Build history of the part. All positions in model axes, mm. Face numbers are marked on the shaded views. Round coordinates to 2 decimals unless told otherwise and drop trailing zeros. Order: outer loops, then holes, each group sorted by start corner. A loop starts at its lowest first (then second) coordinate and runs counter-clockwise, first axis right, second up. Notation, with made-up numbers: (26.5, 0.5) -> (51.5, 0.5) arc R23 ccw to (51.5, 26.5) -> close; hole circle Ø5 at (37.5, 86). An arc over 180 degrees is marked (long way). Use a Markdown table: item, result. Add a question column.
Item 1: Slice it at A-A, the plane z = 0. Give the cut face in (x, y).
Item 2: Probe L1, parallel to Y at x = 30, z = 0; L2, parallel to X at y = -36.5, z = -18; L3, parallel to Z at x = 4, y = -23. List the from-to ranges inside material, lowest first.
Item 3: Two-plate mould, pull along Y, no slides. Class the marked faces 1 and 2: released by +Y, released by -Y, zero draft, split by the parting line, or undercut.
Item 4: Slice it at B-B, the plane y = -29.5. Give the cut face in (x, z), plus the area to 3 significant figures.
Item 5: Pin check, flat tips, straight feed: pin 1 (8 mm diameter, centred on x = 52, y = 28, fed in from +Z); pin 2 (3 mm diameter, centred on x = 39, y = -27, fed in from +Z); pin 3 (6 mm diameter, centred on x = 82, y = -12.5, fed in from +Z); pin 4 (1.5 mm diameter, centred on x = 43.5, y = 32, fed in from -Z). Stop position of each tip, or through.
Item 6: Slice it at C-C, the plane x = 38. Give the cut face in (y, z), plus the area to 3 significant figures.
Item 7: Slice it at D-D, the plane y = 18. Give the cut face in (x, z).
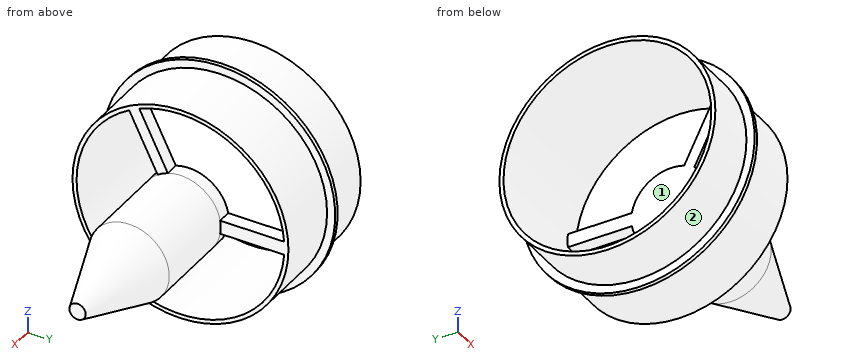
from build123d import *
from build123d.topology import SkipClean

# Parameters (mm, degrees)
SKETCH_1_R          = 39.7
EXTRUDE_1_DEPTH     = 45
SKETCH_2_R          = 38.2
CUT_EXTRUDE_1_DEPTH = 72.952623302
SKETCH_3_R          = 42.7
SKETCH_3_R_2        = 39.7
EXTRUDE_2_DEPTH     = 1.5
EXTRUDE_START       = -5
EXTRUDE_3_DEPTH     = 5
SKETCH_7_R          = 14.8
EXTRUDE_4_DEPTH     = 32.1
SKETCH_9_R          = 14.8
SKETCH_10_R         = 3


with BuildPart() as part:
    # Эскиз1 → Бобышка-Вытянуть1 (new body)
    with BuildSketch(Plane(origin=(0, 0, 0), x_dir=(0, 0, -1), z_dir=(1, 0, 0))):
        with Locations(Location((0, 0, 0), (0, 0, 180))):
            Circle(SKETCH_1_R)
    extrude(amount=EXTRUDE_1_DEPTH)

    # Эскиз2 → Вырез-Вытянуть1 (cut, through all)
    with BuildSketch(Plane.ZY):
        Circle(SKETCH_2_R)
    extrude(amount=-CUT_EXTRUDE_1_DEPTH, mode=Mode.SUBTRACT)

    # Эскиз3 → Бобышка-Вытянуть2 (add)
    with BuildSketch(Plane(origin=(19.4, 0, 0), x_dir=(0, 0, -1), z_dir=(1, 0, 0))):
        Circle(SKETCH_3_R)
        with Locations(Location((0, 0, 0), (0, 0, 180))):
            Circle(SKETCH_3_R_2, mode=Mode.SUBTRACT)
    extrude(amount=EXTRUDE_2_DEPTH)

    # Эскиз6 → Бобышка-Вытянуть3 (add)
    with BuildSketch(Plane(origin=(45, 0, 0), x_dir=(0, 0, -1), z_dir=(1, 0, 0)).offset(EXTRUDE_START)):
        with BuildLine():
            Line((-2.5, 14.587323264), (-2.5, 38.118105934))
            ThreePointArc((-2.5, 38.118105934), (0, 38.2), (2.5, 38.118105934))
            Line((2.5, 38.118105934), (2.5, 14.587323264))
            ThreePointArc((2.5, 14.587323264), (12.69187237, 7.612908495), (14.046441999, -4.662345674))
            Line((14.046441999, -4.662345674), (35.075432195, -15.131227853))
            ThreePointArc((35.075432195, -15.131227853), (34.196736932, -17.024194054), (33.215973901, -18.86634776))
            Line((33.215973901, -18.86634776), (12.186983705, -8.397465581))
            ThreePointArc((12.186983705, -8.397465581), (0, -14.8), (-12.186983705, -8.397465581))
            Line((-12.186983705, -8.397465581), (-33.215973901, -18.86634776))
            ThreePointArc((-33.215973901, -18.86634776), (-34.196736932, -17.024194054), (-35.075432195, -15.131227853))
            Line((-35.075432195, -15.131227853), (-14.046441999, -4.662345674))
            ThreePointArc((-14.046441999, -4.662345674), (-12.69187237, 7.612908495), (-2.5, 14.587323264))
        make_face()
    extrude(amount=EXTRUDE_3_DEPTH)

    # Эскиз7 → Бобышка-Вытянуть4 (add)
    with SkipClean():  # the faces are left unmerged after this step: merging them gives an invalid solid
        with BuildSketch(Plane(origin=(45, 0, 0), x_dir=(0, 0, -1), z_dir=(1, 0, 0))):
            Circle(SKETCH_7_R)
        extrude(amount=EXTRUDE_4_DEPTH)

    # Эскиз9 → По сечениям1 section 0
    with SkipClean():  # the faces are left unmerged after this step: merging them gives an invalid solid
        with BuildSketch(Plane(origin=(77.1, 0, 0), x_dir=(0, 0, -1), z_dir=(1, 0, 0))):
            Circle(SKETCH_9_R)
        # Эскиз10 → По сечениям1 section 1
        with BuildSketch(Plane(origin=(109.2, 0, 0), x_dir=(0, 0, -1), z_dir=(1, 0, 0))):
            Circle(SKETCH_10_R)
        loft()


solid = part.part
Check sheet entries:
| question | item | result |
|---|---|---|
| 1 | outline | (0, -39.7) -> (19.4, -39.7) -> (19.4, -42.7) -> (20.9, -42.7) -> (20.9, -39.7) -> (45, -39.7) -> (45, -38.2) -> (0, -38.2) -> close; (0, 38.2) -> (40, 38.2) -> (40, -14.8) -> (77.1, -14.8) -> (109.2, -3) -> (109.2, 3) -> (77.1, 14.8) -> (45, 14.8) -> (45, 39.7) -> (20.9, 39.7) -> (20.9, 42.7) -> (19.4, 42.7) -> (19.4, 39.7) -> (0, 39.7) -> close |
| 2 | L1 | -39.7 to -38.2, 38.2 to 39.7 |
| 2 | L2 | 19.4 to 20.9 |
| 2 | L3 | -32.36 to -30.5, 30.5 to 32.36 |
| 3 | face 1 | undercut |
| 3 | face 2 | split by the parting line |
| 4 | outline | (0, -26.57) -> (19.4, -26.57) -> (19.4, -30.87) -> (20.9, -30.87) -> (20.9, -26.57) -> (45, -26.57) -> (45, -24.27) -> (0, -24.27) -> close; (0, 24.27) -> (45, 24.27) -> (45, 26.57) -> (20.9, 26.57) -> (20.9, 30.87) -> (19.4, 30.87) -> (19.4, 26.57) -> (0, 26.57) -> close |
| 4 | area | 220 mm2 |
| 5 | pin 1 | through |
| 5 | pin 2 | z = 30.43 |
| 5 | pin 3 | z = 9.26 |
| 5 | pin 4 | z = -24.49 |
| 6 | outline | circle Ø79.4 at (0, 0); hole circle Ø76.4 at (0, 0) |
| 6 | area | 367 mm2 |
| 7 | outline | (0, -35.38) -> (19.4, -35.38) -> (19.4, -38.72) -> (20.9, -38.72) -> (20.9, -35.38) -> (45, -35.38) -> (45, -33.69) -> (0, -33.69) -> close; (0, 33.69) -> (45, 33.69) -> (45, 35.38) -> (20.9, 35.38) -> (20.9, 38.72) -> (19.4, 38.72) -> (19.4, 35.38) -> (0, 35.38) -> close; (40, -2.5) -> (45, -2.5) -> (45, 2.5) -> (40, 2.5) -> close |
